Input: part model. Units: mm. Frame: model coordinates. Coordinates: 2 decimals unless noted, no trailing zeros. Order: outer loops, then holes, each group sorted by start corner. A loop starts at its lowest first (then second) coordinate and runs counter-clockwise, first axis right, second up. Notation, with made-up numbers: (56.5, 59.25) - (87.5, 59.25) arc R23 ccw to (87.5, 88.25) - close; hole circle Ø1 at (-16, 10). An arc over 180 degrees is marked (long way). Use a Markdown table: item, result. Add a question column.
from build123d import *

# Parameters (mm, degrees)
SKETCH1_W           = 150
SKETCH1_H           = 75
BOSS_EXTRUDE1_DEPTH = 3
SKETCH2_R           = 11.11
CUT_EXTRUDE1_DEPTH  = 10


with BuildPart() as part:
    # Sketch1 → Boss-Extrude1 (new body)
    with BuildSketch(Plane.XY):
        with Locations((75, 37.5)):
            Rectangle(SKETCH1_W, SKETCH1_H)
    extrude(amount=BOSS_EXTRUDE1_DEPTH)

    # Sketch2 → Cut-Extrude1 (cut)
    with BuildSketch(Plane.XY.offset(3)):
        with Locations((36.327910431, 59.217033853)):
            Circle(SKETCH2_R)
        with Locations((85.413576885, 13.949141457)):
            Circle(SKETCH2_R)
        with BuildLine():
            Line((17.12526901, 7.718435361), (17.12526901, 17.718435361))
            ThreePointArc((17.12526901, 17.718435361), (19.87526901, 20.468435361), (22.62526901, 17.718435361))
            Line((22.62526901, 17.718435361), (22.62526901, 7.718435361))
            ThreePointArc((22.62526901, 7.718435361), (19.87526901, 4.968435361), (17.12526901, 7.718435361))
        make_face()
        with BuildLine():
            Line((41.656612513, 7.718435361), (41.656612513, 17.718435361))
            ThreePointArc((41.656612513, 17.718435361), (44.406612513, 20.468435361), (47.156612513, 17.718435361))
            Line((47.156612513, 17.718435361), (47.156612513, 7.718435361))
            ThreePointArc((47.156612513, 7.718435361), (44.406612513, 4.968435361), (41.656612513, 7.718435361))
        make_face()
    extrude(amount=-CUT_EXTRUDE1_DEPTH, mode=Mode.SUBTRACT)


solid = part.part
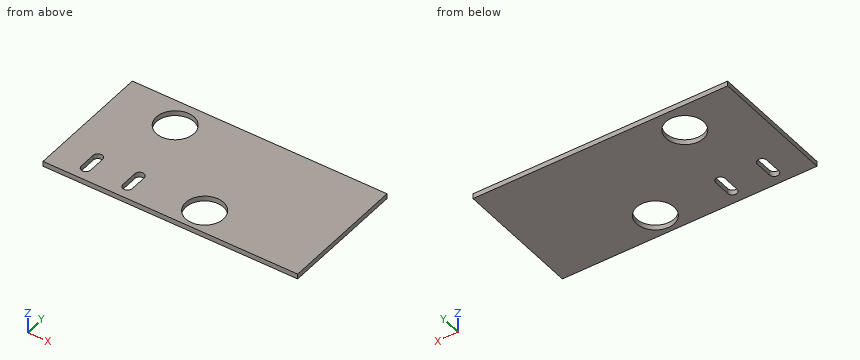
1) Cut plane B-B (z = 1.5). Return the cut outline in (x, y).
2) Contact query for a flat-ended pin moving along its axis: P1, Ø20, axis at x = 36.33, y = 59.22, coming from the +Z side. Output: stop coordinate, or through.
3) Material intervals for L1, parallel to X at y = 17.5, z = 0.55; L2, parallel to X at y = 55.5, z = 2.65; L3, parallel to X at y = 5.5, z = 2.9, sorted ascending.
4) Cut plane A-A (x = 34). Return the cut outline in (y, z).
Computed:
| question | item | result |
|---|---|---|
| 1 | outline | (0, 0) - (150, 0) - (150, 75) - (0, 75) - close; hole (17.13, 7.72) arc R2.75 ccw to (22.63, 7.72) - (22.63, 17.72) arc R2.75 ccw to (17.13, 17.72) - close; hole circle Ø22.22 at (36.33, 59.22); hole (41.66, 7.72) arc R2.75 ccw to (47.16, 7.72) - (47.16, 17.72) arc R2.75 ccw to (41.66, 17.72) - close; hole circle Ø22.22 at (85.41, 13.95) |
| 2 | P1 | passes through |
| 3 | L1 | x = 0 to 17.13, 22.63 to 41.66, 47.16 to 74.89, 95.94 to 150 |
| 3 | L2 | x = 0 to 25.86, 46.8 to 150 |
| 3 | L3 | x = 0 to 18.25, 21.5 to 42.78, 46.03 to 78.2, 92.63 to 150 |
| 4 | outline | (0, 0) - (48.35, 0) - (48.35, 3) - (0, 3) - close; (70.08, 0) - (75, 0) - (75, 3) - (70.08, 3) - close |
